The model under review builds one solid part; all positions refer to its coordinate system, in mm. Face numbers are marked on the shaded views. A direction names the side the tool comes from. Coordinates: 2 decimals unless noted, no trailing zeros. Order: outer loops, then holes, each group sorted by start corner. A loop starts at its lowest first (then second) coordinate and runs counter-clockwise, first axis right, second up. Notation, with made-up numbers: (-32.75, 58) -> (10.25, 58) arc R11 ccw to (10.25, 69) -> close; hole circle Ø4 at (-7, -6.5). An arc over 180 degrees is marked (long way). Use CSV: the item, a comma, the result in double quotes. Start each with the question number.
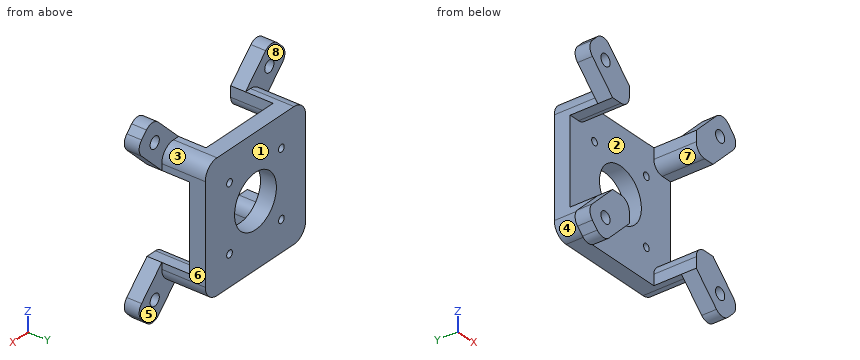
```python
from build123d import *

# Parameters (mm, degrees)
SKETCH2_W           = 60
SKETCH2_H           = 60
SKETCH2_R           = 1.7
SKETCH2_R_2         = 12.5
BOSS_EXTRUDE2_DEPTH = 7.5
SKETCH3_W           = 10
SKETCH3_H           = 10
BOSS_EXTRUDE3_DEPTH = 20
BOSS_EXTRUDE5_DEPTH = 7
FILLET2_R           = 7
FILLET3_R           = 5
SKETCH7_R           = 2.75
CUT_EXTRUDE1_DEPTH  = 68.430967848


with BuildPart() as part:
    # Sketch2 → Boss-Extrude2 (new body)
    with BuildSketch(Plane(origin=(0, 0, 0), x_dir=(1, 0, 0), z_dir=(0, 1, 0))):
        Rectangle(SKETCH2_W, SKETCH2_H)
        with Locations(Location((-15.5, 15.5, 0), (0, 0, 270))):
            Circle(SKETCH2_R, mode=Mode.SUBTRACT)
        with Locations(Location((15.5, 15.5, 0), (0, 0, 90))):
            Circle(SKETCH2_R, mode=Mode.SUBTRACT)
        with Locations(Location((-15.5, -15.5, 0), (0, 0, 90))):
            Circle(SKETCH2_R, mode=Mode.SUBTRACT)
        with Locations(Location((15.5, -15.5, 0), (0, 0, 270))):
            Circle(SKETCH2_R, mode=Mode.SUBTRACT)
        with Locations(Location((0, 0, 0), (0, 0, 270))):
            Circle(SKETCH2_R_2, mode=Mode.SUBTRACT)
    extrude(amount=BOSS_EXTRUDE2_DEPTH)

    # Sketch3 → Boss-Extrude3 (add)
    with BuildSketch(Plane.XZ):
        with Locations((-25, 25)):
            Rectangle(SKETCH3_W, SKETCH3_H)
        with Locations((-25, -25)):
            Rectangle(SKETCH3_W, SKETCH3_H)
        with Locations((25, -25)):
            Rectangle(SKETCH3_W, SKETCH3_H)
        with Locations((25, 25)):
            Rectangle(SKETCH3_W, SKETCH3_H)
    extrude(amount=BOSS_EXTRUDE3_DEPTH)

    # Sketch5 → Boss-Extrude5 (add)
    with BuildSketch(Plane.XZ.offset(20)):
        with BuildLine():
            Line((20, -30), (32.071067812, -42.071067812))
            ThreePointArc((32.071067812, -42.071067812), (35.606601718, -43.535533906), (39.142135624, -42.071067812))
            Line((39.142135624, -42.071067812), (42.071067812, -39.142135624))
            ThreePointArc((42.071067812, -39.142135624), (43.535533906, -35.606601718), (42.071067812, -32.071067812))
            Line((42.071067812, -32.071067812), (30, -20))
            Line((30, -20), (20, -20))
            Line((20, -20), (20, -30))
        make_face()
        with BuildLine():
            Line((-20, -20), (-20, -30))
            Line((-20, -30), (-32.071067812, -42.071067812))
            ThreePointArc((-32.071067812, -42.071067812), (-35.606601718, -43.535533906), (-39.142135624, -42.071067812))
            Line((-39.142135624, -42.071067812), (-42.071067812, -39.142135624))
            ThreePointArc((-42.071067812, -39.142135624), (-43.535533906, -35.606601718), (-42.071067812, -32.071067812))
            Line((-42.071067812, -32.071067812), (-30, -20))
            Line((-30, -20), (-20, -20))
        make_face()
        with BuildLine():
            Line((20, 20), (20, 30))
            Line((20, 30), (32.071067812, 42.071067812))
            ThreePointArc((32.071067812, 42.071067812), (35.606601718, 43.535533906), (39.142135624, 42.071067812))
            Line((39.142135624, 42.071067812), (42.071067812, 39.142135624))
            ThreePointArc((42.071067812, 39.142135624), (43.535533906, 35.606601718), (42.071067812, 32.071067812))
            Line((42.071067812, 32.071067812), (30, 20))
            Line((30, 20), (20, 20))
        make_face()
        with BuildLine():
            Line((-20, 30), (-32.071067812, 42.071067812))
            ThreePointArc((-32.071067812, 42.071067812), (-35.606601718, 43.535533906), (-39.142135624, 42.071067812))
            Line((-39.142135624, 42.071067812), (-42.071067812, 39.142135624))
            ThreePointArc((-42.071067812, 39.142135624), (-43.535533906, 35.606601718), (-42.071067812, 32.071067812))
            Line((-42.071067812, 32.071067812), (-30, 20))
            Line((-30, 20), (-20, 20))
            Line((-20, 20), (-20, 30))
        make_face()
    extrude(amount=-BOSS_EXTRUDE5_DEPTH)

    # Fillet2
    fillet2_edges = [part.edges().sort_by_distance(p)[0] for p in [
        (30, -2.75, 30),
        (-30, -2.75, 30),
        (-30, -2.75, -30),
        (30, -2.75, -30),
    ]]
    fillet(fillet2_edges, radius=FILLET2_R)

    # Fillet3
    fillet3_edges = [part.edges().sort_by_distance(p)[0] for p in [
        (-20, -10, 20),
        (-20, -10, -20),
        (20, -10, -20),
        (20, -10, 20),
    ]]
    fillet(fillet3_edges, radius=FILLET3_R)

    # Sketch7 → Cut-Extrude1 (cut, through all)
    with BuildSketch(Plane.XZ.offset(20)):
        with Locations(Location((34.242640687, -34.242640687, 0), (0, 0, 270))):
            Circle(SKETCH7_R)
        with Locations(Location((-34.242640687, -34.242640687, 0), (0, 0, 270))):
            Circle(SKETCH7_R)
        with Locations(Location((-34.242640687, 34.242640687, 0), (0, 0, 270))):
            Circle(SKETCH7_R)
        with Locations(Location((34.242640687, 34.242640687, 0), (0, 0, 270))):
            Circle(SKETCH7_R)
    extrude(amount=-CUT_EXTRUDE1_DEPTH, mode=Mode.SUBTRACT)


solid = part.part
```
Q1. Draft analysis for pull direction X (two halves, no side actions). For the marked faces 1, 2, 3 and 4, state which applies: +X half, -X half, draft (parallel to the pull), parting line (faces both ways), or undercut.
Q2. To check wall thickness, follow probe 1 along X at (y, z) = (5.5, 15.5); probe 2 along Z at (x, y) = (15, 0.25); probe 3 along Y at (x, z) = (13, -20). State the ranges of each line that lie inside material, in increasing order.
Q3. For the marked faces 5, 6, 7 and 8, list the 3-axis set-ups (+Z, -Z, +X, -X, +Y, -Y) from which the entire face can be reached by the end or side of a thin tool; tool diameter is ignored.
Q4. Add section C-C, the plane z = 0.5. State the section outline as (x, y) points, then the cut area to 3 significant figures.
Q5. Add section A-A, the plane y = -11.5. State the section outline as (x, z) points, then the cut area to 3 significant figures.
Q6. Add section B-B, the plane z = -15.5. State the section outline as (x, y) points, then the cut area to 3 significant figures.
Q7. Add section D-D, the plane x = 15.5. State the section outline as (y, z) points.
Q8. Clearance check with flat-ended pins moving along their axes: pin 1 Ø7 at (x, z) = (-35, -32) entering from +Y; pin 2 Ø5 at (x, z) = (34.24, 34.24) entering from +Y; pin 3 Ø2.5 at (y, z) = (-14, 26.5) entering from +X; pin 4 Ø1.5 at (x, y) = (26.5, -5) entering from +Z. State where each tip first meets the part, or that it passes through.
Answer block:
1,face 1,"draft"
1,face 2,"undercut"
1,face 3,"+X half"
1,face 4,"-X half"
2,probe 1,"x = -30 to -17.2, -13.8 to 13.8, 17.2 to 30"
2,probe 2,"z = -30 to -17.12, -13.88 to 13.88, 17.12 to 30"
2,probe 3,"y = 0 to 7.5"
3,face 5,"-Z, +X, +Y"
3,face 6,"+Z, -Z, +X, +Y"
3,face 7,"-Y"
3,face 8,"+Z, -X, +Y"
4,outline,"(-30, 0) -> (-12.49, 0) -> (-12.49, 7.5) -> (-30, 7.5) -> close; (12.49, 0) -> (30, 0) -> (30, 7.5) -> (12.49, 7.5) -> close"
4,area,"263 mm²"
5,outline,"(-30, -23) arc R7 ccw to (-23, -30) -> (-20, -30) -> (-20, -25) arc R5 ccw to (-25, -20) -> (-30, -20) -> close; (-30, 20) -> (-25, 20) arc R5 ccw to (-20, 25) -> (-20, 30) -> (-23, 30) arc R7 ccw to (-30, 23) -> close; (20, -30) -> (23, -30) arc R7 ccw to (30, -23) -> (30, -20) -> (25, -20) arc R5 ccw to (20, -25) -> close; (20, 25) arc R5 ccw to (25, 20) -> (30, 20) -> (30, 23) arc R7 ccw to (23, 30) -> (20, 30) -> close"
5,area,"336 mm²"
6,outline,"(-30, 0) -> (-17.2, 0) -> (-17.2, 7.5) -> (-30, 7.5) -> close; (-13.8, 0) -> (13.8, 0) -> (13.8, 7.5) -> (-13.8, 7.5) -> close; (17.2, 0) -> (30, 0) -> (30, 7.5) -> (17.2, 7.5) -> close"
6,area,"399 mm²"
7,outline,"(0, -30) -> (7.5, -30) -> (7.5, -17.2) -> (0, -17.2) -> close; (0, -13.8) -> (7.5, -13.8) -> (7.5, 13.8) -> (0, 13.8) -> close; (0, 17.2) -> (7.5, 17.2) -> (7.5, 30) -> (0, 30) -> close"
8,pin 1,"stops at y = -13"
8,pin 2,"passes through"
8,pin 3,"stops at x = 37.75"
8,pin 4,"stops at z = 29.44"
